Check sheet for the drawn part. Datum: minimum x, y, z corner. Units: mm. A direction names the side the tool comes from. Round coordinates to 2 decimals unless told otherwise and drop trailing zeros. Write each loop counter-clockwise with the first axis right and the second up, starting at its lowest first coordinate (ties: lowest second). Pieces come first, ordered by that corner, then holes. Notation, with made-up numbers: (68, 68.25) - (117, 68.25) arc R31 ccw to (117, 97.25) - close; hole circle Ø9 at (-28.5, 68). An arc over 180 degrees is marked (long way). Answer as a JSON object with one key per item and string values.
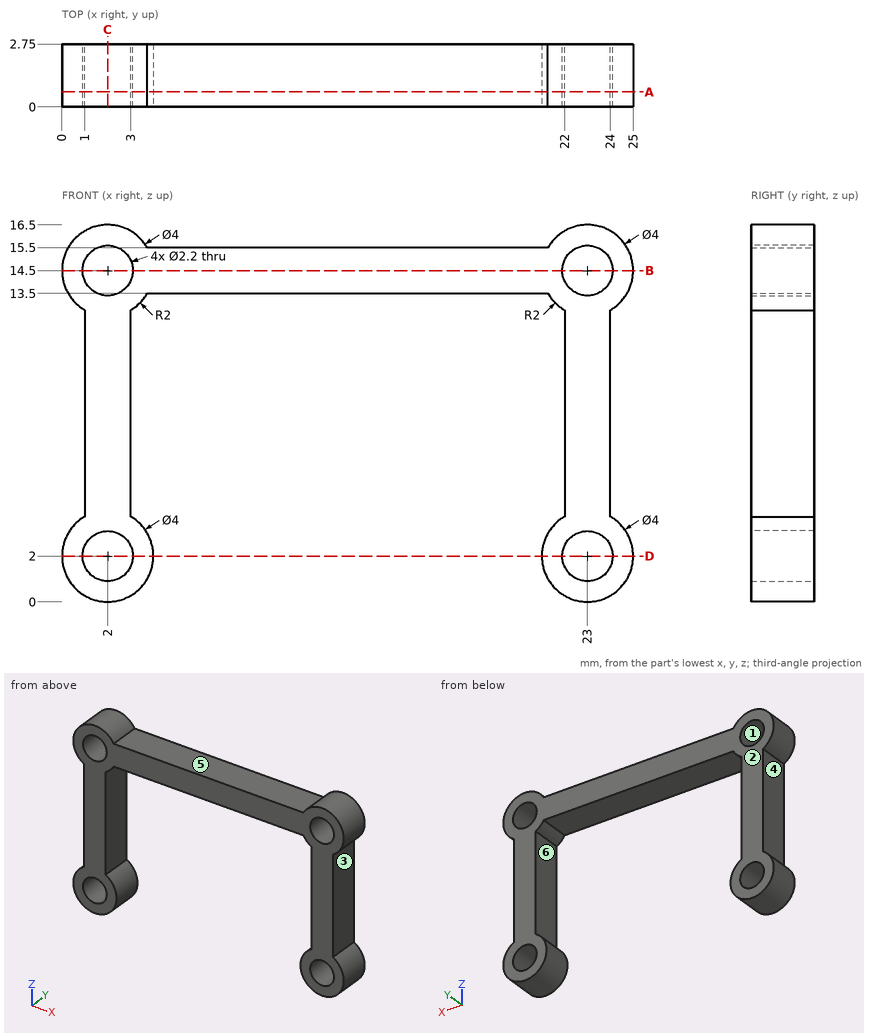
1. Go/stop test with flat-tipped pins: pin 1 (1.4 mm diameter, centred on y = 1, z = 7.5, fed in from -X); pin 2 (3 mm diameter, centred on x = 23, z = 14.5, fed in from +Y); pin 3 (1.3 mm diameter, centred on x = 23, z = 2, fed in from +Y); pin 4 (1.5 mm diameter, centred on x = 14.5, y = 0.5, fed in from -Z). Record where each tip stops, or that it passes through.
Completed:
{"pin 1": "stops at x = 1", "pin 2": "stops at y = 2.75", "pin 3": "passes through", "pin 4": "stops at z = 13.5"}
2. Cross-section at C-C (x = 2). Record the boundary of the cut face in (y, z), plus the area to 3 significant figures.
Completed:
{"outline": "(0, 0) - (2.75, 0) - (2.75, 0.9) - (0, 0.9) - close; (0, 3.1) - (2.75, 3.1) - (2.75, 13.4) - (0, 13.4) - close; (0, 15.6) - (2.75, 15.6) - (2.75, 16.5) - (0, 16.5) - close", "area": "33.3 mm^2"}
3. Material ranges on probe 1 along X at (y, z) = (1.1, 14.5); probe 2 along X at (y, z) = (2.15, 8.5); probe 3 along Z at (x, y) = (22.75, 1.2), recorded low to high. Write a range as from..to.
Completed:
{"probe 1": "x = 0..0.9, 3.1..21.9, 24.1..25", "probe 2": "x = 1..3, 22..24", "probe 3": "z = 0.02..0.93, 3.07..13.43, 15.57..16.48"}
4. Cross-section at B-B (z = 14.5). Record the boundary of the cut face in (x, y).
Completed:
{"outline": "(0, 0) - (0.9, 0) - (0.9, 2.75) - (0, 2.75) - close; (3.1, 0) - (21.9, 0) - (21.9, 2.75) - (3.1, 2.75) - close; (24.1, 0) - (25, 0) - (25, 2.75) - (24.1, 2.75) - close"}
5. Cross-section at A-A (y = 0.65). Record the boundary of the cut face in (x, z).
Completed:
{"outline": "(1, 3.73) arc R2 ccw (long way) to (3, 3.73) - (3, 12.77) arc R2 ccw to (3.73, 13.5) - (21.27, 13.5) arc R2 ccw to (22, 12.77) - (22, 3.73) arc R2 ccw (long way) to (24, 3.73) - (24, 12.77) arc R2 ccw (long way) to (21.27, 15.5) - (3.73, 15.5) arc R2 ccw (long way) to (1, 12.77) - close; hole circle Ø2.2 at (2, 2); hole circle Ø2.2 at (2, 14.5); hole circle Ø2.2 at (23, 2); hole circle Ø2.2 at (23, 14.5)"}
6. Mould release check, pull along X, two halves, no side actions. Record for the marked faces 1, 2 and 3: released by +X, released by -X, zero draft, split by the parting line, or undercut.
Completed:
{"face 1": "undercut", "face 2": "zero draft", "face 3": "released by +X"}
7. Access from +Z, -Z, +X, -X, +Y, -Y to the whole of each face (thin tool, end or side, straight path). Record for the marked faces 4, 5 and 6.
Completed:
{"face 4": "-X, +Y, -Y", "face 5": "+Z, +Y, -Y", "face 6": "+Y, -Y"}
8. Cross-section at D-D (z = 2). Record the boundary of the cut face in (x, y).
Completed:
{"outline": "(0, 0) - (0.9, 0) - (0.9, 2.75) - (0, 2.75) - close; (3.1, 0) - (4, 0) - (4, 2.75) - (3.1, 2.75) - close; (21, 0) - (21.9, 0) - (21.9, 2.75) - (21, 2.75) - close; (24.1, 0) - (25, 0) - (25, 2.75) - (24.1, 2.75) - close"}
